CAD build for the part. Positions are in the model's coordinates, mm. A direction names the side the tool comes from. Round coordinates to 2 decimals unless told otherwise and drop trailing zeros. Loops run counter-clockwise (first coordinate to the right, second up) from the corner with the lowest first, then second, coordinate; pieces in that order, holes last. Notation, with made-up numbers: M -14,-3.75 L 15,-3.75 A25 ccw 15,26.25 Z; hole C 18.25,-38 d8. An arc over 180 degrees is marked long. Use one line per item in the form item = value.
from build123d import *

# Parameters (mm, degrees)
SKETCH1_W          = 21.3
SKETCH1_H          = 13.02
EXTRUDE1_DEPTH     = 7.25
CUT_EXTRUDE1_DEPTH = 0.127
CUT_EXTRUDE2_DEPTH = 11.303
EXTRUDE2_DEPTH     = 3.79984
CUT_EXTRUDE3_START = -11.43
SKETCH5_W          = 0.44704
SKETCH5_H          = 3.302
CUT_EXTRUDE3_DEPTH = 8.89
EXTRUDE3_DEPTH     = 2.7051
EXTRUDE4_DEPTH     = 0.381


with BuildPart() as part:
    # Sketch1 → Extrude1 (new, symmetric)
    with BuildSketch(Plane(origin=(0, 0, 0), x_dir=(0, 0, -1), z_dir=(1, 0, 0))):
        with Locations((-10.65, 6.51)):
            Rectangle(SKETCH1_W, SKETCH1_H)
    extrude(amount=EXTRUDE1_DEPTH, both=True)

    # Sketch2 → Cut-Extrude1 (cut)
    with BuildSketch(Plane.XY.offset(21.3)):
        Polygon((-5.9436, 11.43), (5.9436, 11.43), (5.9436, 1.0668), (2.9718, 1.0668), (2.9718, 0), (-2.9718, 0), (-2.9718, 1.0668), (-5.9436, 1.0668), align=None)
    extrude(amount=-CUT_EXTRUDE1_DEPTH, mode=Mode.SUBTRACT)

    # Sketch3 → Cut-Extrude2 (cut)
    with BuildSketch(Plane.XY.offset(21.173)):
        Polygon((-5.9436, 3.0988), (-3.2004, 3.0988), (-3.2004, 1.0668), (3.2004, 1.0668), (3.2004, 3.0988), (5.9436, 3.0988), (5.9436, 11.43), (-5.9436, 11.43), align=None)
    extrude(amount=-CUT_EXTRUDE2_DEPTH, mode=Mode.SUBTRACT)

    # Sketch4 → Extrude2 (add, symmetric)
    with BuildSketch(Plane(origin=(0, 0, 0), x_dir=(0, 0, -1), z_dir=(1, 0, 0))):
        Polygon((-17.592809528, 11.43), (-18.76, 11.43), (-9.87, 8.128), (-9.87, 8.56152789), align=None)
    extrude(amount=EXTRUDE2_DEPTH, both=True)

    # Sketch5 → Cut-Extrude3 (cut)
    with BuildSketch(Plane.XY.offset(21.3).offset(CUT_EXTRUDE3_START)):
        with Locations((-3.12928, 9.779)):
            Rectangle(SKETCH5_W, SKETCH5_H)
        with Locations((-2.2352, 9.779)):
            Rectangle(SKETCH5_W, SKETCH5_H)
        with Locations((-1.34112, 9.779)):
            Rectangle(SKETCH5_W, SKETCH5_H)
        with Locations((-0.44704, 9.779)):
            Rectangle(SKETCH5_W, SKETCH5_H)
        with Locations((0.44704, 9.779)):
            Rectangle(SKETCH5_W, SKETCH5_H)
        with Locations((1.34112, 9.779)):
            Rectangle(SKETCH5_W, SKETCH5_H)
        with Locations((2.2352, 9.779)):
            Rectangle(SKETCH5_W, SKETCH5_H)
        with Locations((3.12928, 9.779)):
            Rectangle(SKETCH5_W, SKETCH5_H)
    extrude(amount=CUT_EXTRUDE3_DEPTH, mode=Mode.SUBTRACT)

    # Sketch6 → Extrude3 (add)
    with BuildSketch(Plane(origin=(-5.9436, 0, 0), x_dir=(0, 0, -1), z_dir=(1, 0, 0))):
        Polygon((-9.87, 3.0988), (-21.082, 3.0988), (-20.3708, 3.81), (-12.446, 3.81), (-12.446, 4.826), (-9.87, 4.826), align=None)
    extrude3 = extrude(amount=EXTRUDE3_DEPTH)

    # Mirror1: Extrude3 across plane
    add(extrude3.mirror(Plane(origin=(0, 0, 0), x_dir=(0, 0, 1), z_dir=(1, 0, 0))))

    # Sketch14 → Extrude4 (add)
    with BuildSketch(Plane.XZ):
        Polygon((-6.604, 21.3), (-2.9718, 21.3), (-2.9718, 20.792), (2.9718, 20.792), (2.9718, 21.3), (6.604, 21.3), (6.604, 18.252), (-6.604, 18.252), align=None)
    extrude(amount=EXTRUDE4_DEPTH)


solid = part.part
1. Probe line 1 along X through (y, z) = (1.75, 11); line 2 along X through (y, z) = (8.5, 17); line 3 along Y through (x, z) = (-3.5, 16.75). List the from-to ranges inside material, lowest first. Write a range as from..to.
Completed:
line_1 = -7.25..-3.2, 3.2..7.25
line_2 = -7.25..-5.94, 5.94..7.25
line_3 = 0..3.81, 10.68..11.12, 11.43..13.02
2. Tool access for faces 3 (the face through (-0.891, 9.976, 13.677)), 4 (the face through (-3.353, 9.9, 14)): list every direction of +Z, -Z, +X, -X, +Y, -Y with a clear straight run to the whole face (end or side of a thin tool).
Completed:
face_3 = none
face_4 = +Z
3. Pull direction X, two halves, no side cores. Call faces 1 (the face through (-2.459, 9.9, 14)), 2 (the face through (7.25, 7, 11)): +X half, -X half, draft (parallel to the pull), parting line (faces both ways), or undercut.
Completed:
face_1 = undercut
face_2 = +X half
4. Cut at D-D on z = 7. Write the cut outline in (x, y).
Completed:
outline = M -7.25,0 L 7.25,0 L 7.25,13.02 L -7.25,13.02 Z
5. Cut at A-A on x = -4.75. Write the cut outline in (y, z).
Completed:
outline = M -0.38,18.25 L 0,18.25 L 0,0 L 13.02,0 L 13.02,21.3 L 11.43,21.3 L 11.43,9.87 L 4.83,9.87 L 4.83,12.45 L 3.81,12.45 L 3.81,20.37 L 3.1,21.08 L 3.1,21.17 L 1.07,21.17 L 1.07,21.3 L -0.38,21.3 Z
6. Cut at C-C on z = 14.75. State how many separate pieces and enclosed holes the cut face has, and give its area (3 significant figures).
Completed:
separate_pieces = 10
enclosed_holes = 1
area = 82.3 mm2
7. Cut at B-B on y = 6.5. Write the cut outline in (x, z).
Completed:
outline = M -7.25,0 L 7.25,0 L 7.25,21.3 L 5.94,21.3 L 5.94,9.87 L -5.94,9.87 L -5.94,21.3 L -7.25,21.3 Z
